Verification items for the finished model (mm, model axes). Give positions to 0.01 mm unless a question says otherwise; leave off trailing zeros. Order: outer loops, then holes, each group sorted by start corner. A loop starts at its lowest first (then second) coordinate and runs counter-clockwise, first axis right, second up.
from build123d import *

# Parameters (mm, degrees)
SKETCH1_W           = 10
SKETCH1_H           = 10
SKETCH1_W_2         = 8
SKETCH1_H_2         = 8
BOSS_EXTRUDE1_DEPTH = 542
SKETCH2_R           = 2.125
CUT_EXTRUDE1_DEPTH  = 116
SKETCH3_R           = 2.1
SKETCH3_R_2         = 2.125
CUT_EXTRUDE2_DEPTH  = 10
SKETCH5_R           = 2.125
CUT_EXTRUDE3_DEPTH  = 10


with BuildPart() as part:
    # Sketch1 → Boss-Extrude1 (new body)
    with BuildSketch(Plane.XY):
        with Locations((5, 5)):
            Rectangle(SKETCH1_W, SKETCH1_H)
        with Locations((5, 5)):
            Rectangle(SKETCH1_W_2, SKETCH1_H_2, mode=Mode.SUBTRACT)
    extrude(amount=BOSS_EXTRUDE1_DEPTH)

    # Sketch2 → Cut-Extrude1 (cut)
    with BuildSketch(Plane(origin=(0, 10, 0), x_dir=(1, 0, 0), z_dir=(0, 1, 0))):
        with Locations(Location((5, -5, 0), (0, 0, 270))):
            Circle(SKETCH2_R)
        with Locations(Location((5, -15, 0), (0, 0, 270))):
            Circle(SKETCH2_R)
        with Locations(Location((5, -527, 0), (0, 0, 270))):
            Circle(SKETCH2_R)
        with Locations(Location((5, -537, 0), (0, 0, 270))):
            Circle(SKETCH2_R)
    extrude(amount=-CUT_EXTRUDE1_DEPTH, mode=Mode.SUBTRACT)

    # Sketch3 → Cut-Extrude2 (cut)
    with BuildSketch(Plane.XZ):
        with Locations(Location((5, 326, 0), (0, 0, 270))):
            Circle(SKETCH3_R)
        with Locations(Location((5, 226, 0), (0, 0, 270))):
            Circle(SKETCH3_R_2)
    extrude(amount=-CUT_EXTRUDE2_DEPTH, mode=Mode.SUBTRACT)

    # Sketch5 → Cut-Extrude3 (cut)
    with BuildSketch(Plane(origin=(10, 0, 0), x_dir=(0, 0, -1), z_dir=(1, 0, 0))):
        with Locations(Location((-447, 5, 0), (0, 0, 90))):
            Circle(SKETCH5_R)
        with Locations(Location((-95, 5, 0), (0, 0, 90))):
            Circle(SKETCH5_R)
        with Locations(Location((-271, 5, 0), (0, 0, 90))):
            Circle(SKETCH5_R)
    extrude(amount=-CUT_EXTRUDE3_DEPTH, mode=Mode.SUBTRACT)


solid = part.part
(1) Section check A-A, the plane z = 457.5. Enter the section's corners in (x, y), then the cut area to 3 significant figures.
Solved:
outline: (0, 0) - (10, 0) - (10, 10) - (0, 10) - close; hole (1, 1) - (9, 1) - (9, 9) - (1, 9) - close
area: 36.0 mm2
(2) Section check B-B, the plane y = 4.5. Give the number of separate pieces and of enclosed holes in the cut face, then the cut area to 3 significant figures.
Solved:
separate pieces: 8
enclosed holes: 0
area: 1,060 mm2
(3) Go/stop test with a flat-tipped pin: pin 1 (2.5 mm diameter, centred on x = 5, z = 5, fed in from -Y). Record where the tip stops, or that it passes through.
Solved:
pin 1: passes through
(4) Scan lines: line 1 (X direction, y = 5.5, z = 441); line 2 (Z direction, x = 9.8, y = 5) (3 decimals). Record each from-to range of solid material in increasing order.
Solved:
line 1: x = 0 to 1, 9 to 10
line 2: z = 0 to 92.875, 97.125 to 268.875, 273.125 to 444.875, 449.125 to 542
